Autodesk Inventor part; units mm, degrees
ref_plane "YZ Plane" through (0, 0, 0) normal (1, 0, 0) x (0, 1, 0)
ref_plane "XZ Plane" through (0, 0, 0) normal (0, 1, 0) x (-1, 0, 0)
ref_plane "XY Plane" through (0, 0, 0) normal (0, 0, 1) x (1, 0, 0)
sketch "Szkic1" plane through (0, 0, 0) normal (1, 0, 0) x (0, 1, 0)
  line L0 (0, 0) -> (50, 0)
  line L1 (50, 0) -> (50, -75)
  line L2 (50, -75) -> (0, -75)
  line L3 (0, -75) -> (0, 0)
  circle A0 centre (75, -37.5) radius 20
  line L4 (50, 0) -> (84.9897, -20.1735)
  line L5 (50, -75) -> (84.9897, -54.8265)
  dimension "d0" = 50
  dimension "d1" = 75
  dimension "d2" = 40
  dimension "d3" = 25
  dimension "d4" = 37.5
extrude "Wyciągnięcie proste1" add sketch "Szkic1" along normal blind 12
sketch "Szkic2" plane through (12, 0, 0) normal (1, 0, 0) x (0, 0, -1)
  point P0 (0, 0)
sketch "Szkic3" plane through (0, 0, 0) normal (-1, 0, 0) x (0, 0, 1)
  arc A0 (-20.1735, 84.9897) -> (-54.8265, 84.9897) centre (-37.5, 75) ccw
  circle A1 centre (-37.5, 75) radius 20
  point P0 (0, 0)
  point P1 (-54.8265, 84.9897)
  point P2 (-20.1735, 84.9897)
  dimension "d7" = 40
extrude "Wyciągnięcie proste2" add sketch "Szkic3" along normal blind 8
sketch "Szkic4" plane through (0, 0, 0) normal (-1, 0, 0) x (0, 0, 1)
  circle A0 centre (-38, 34) radius 8
  circle A1 centre (-38, 20) radius 8
  line L0 (-46, 34) -> (-46, 20)
  line L1 (-30, 34) -> (-30, 20)
  line L2 (0, 0) -> (-75, 0)
  dimension "d10" = 16
  dimension "d11" = 16
  dimension "d12" = 14
  dimension "d13" = 20
extrude "Wyciągnięcie proste3" cut sketch "Szkic4" against normal through all
sketch "Szkic5" plane through (-8, 75, -37.5) normal (-1, 0, 0) x (0, 0, 1)
  point P0 (37.5, -75)
  point P1 (0, 0)
hole "Otwór1" at (-8, 75, -37.5) direction (1, 0, 0) diameter 20 end through all
ref_plane "Płaszczyzna konstrukcyjna1" through (0, 0, -63.5) normal (0, 0, -1) x (-1, 0, 0)
sketch "Szkic6" plane through (0, 0, -63.5) normal (0, 0, -1) x (-1, 0, 0)
  circle A0 centre (20, 12.5) radius 12.5
  line L0 (0, 50) -> (-12, 50)
  line L1 (0, 50) -> (28.8115, 21.3661)
  line L2 (0, 0) -> (0, 50)
  line L3 (0, 0) -> (20, 0)
  dimension "d24" = 25
  dimension "d25" = 20
extrude "Wyciągnięcie proste4" add sketch "Szkic6" against normal blind 10
ref_plane "Płaszczyzna konstrukcyjna2" through (0, 0, -37.5) normal (0, 0, -1) x (-1, 0, 0)
sketch "Szkic7" plane through (0, 0, -63.5) normal (0, 0, -1) x (-1, 0, 0)
  arc A0 (20, 0) -> (28.8115, 21.3661) centre (20, 12.5) ccw
  circle A1 centre (20, 12.5) radius 12.5
  point P0 (0, 0)
  dimension "d28" = 25
extrude "Wyciągnięcie proste5" add sketch "Szkic7" along normal blind 2
sketch "Szkic8" plane through (-20, 12.5, -65.5) normal (0, 0, -1) x (-1, 0, 0)
  point P0 (-20, -12.5)
  point P1 (0, 0)
hole "Otwór2" at (-20, 12.5, -65.5) direction (0, 0, 1) diameter 12 end through all
mirror "Odbij1" about plane through (0, 0, -37.5) normal (0, 0, -1) of "Wyciągnięcie proste4", "Wyciągnięcie proste5", "Otwór2"
fillet "Zaokrąglenie1" radius 1 4 edges at (0, 25, -63.5) (0, 25, -21.5) (0, 25, -11.5) (0, 25, -53.5)
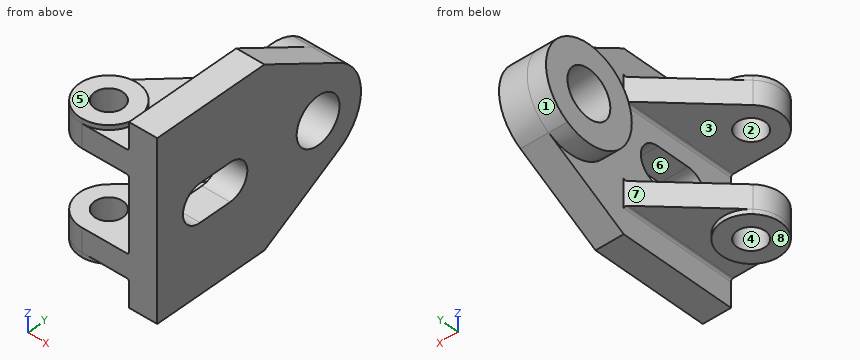
Geometry check sheet. Reference: the model listing, model coordinates, mm. Face numbers are marked on the shaded views. A direction names the side the tool comes from. Coordinates: 2 decimals unless noted, no trailing zeros. Order: outer loops, then holes, each group sorted by start corner. A loop starts at its lowest first (then second) coordinate and runs counter-clockwise, first axis right, second up. Notation, with made-up numbers: (57, 26.25) - (112, 26.25) arc R31 ccw to (112, 59.25) - close; hole circle Ø4 at (45, -39.5). An arc over 180 degrees is marked (long way). Answer in a Markdown table with one row per item. Add a question column.
1) Cross-section at C-C, the plane y = 79. Record the cut outline in (x, z).
2) Material ranges on line 1 along Y through (x, z) = (5.25, -37.5); line 2 along X through (y, z) = (12.5, -15.5); line 3 along Z through (x, y) = (8, 29.5), recorded low to high. Write a range as [from, to].
3) Cross-section at A-A, the plane z = -37.5. Record the cut outline in (x, y), then the cut area to 3 significant figures.
4) Cross-section at B-B, the plane x = -6. Record the cut outline in (y, z), then the cut area to 3 significant figures.
5) Release check for a two-part mould opening along Y. For the marked faces 1, 2, 3 and 4 record: +Y half, -Y half, draft (parallel to the pull), parting line (faces both ways), or undercut.
6) Gauge pin test, flat ends, axial feed: P1, Ø7.5, axis at x = -23.5, y = 8.5, coming from the -Z side; P2, Ø1.5, axis at x = -4.5, z = -10, coming from the -Y side; P3, Ø1.5, axis at x = -2.5, y = 27, coming from the -Z side; P4, Ø22.5, axis at y = 61.5, z = -55, coming from the -X side. Record the tip position at first contact, or that the pin passes through.
7) Cross-section at D-D, the plane x = -23. Record the cut outline in (y, z), then the cut area to 3 significant figures.
8) Set-up check for the marked faces 5, 6, 7 and 8: record each of +Z, -Z, +X, -X, +Y, -Y from which the full face is reachable in a straight line by a thin tool's end or side.
Check result:
| question | item | result |
|---|---|---|
| 1 | outline | (-8, -57.1) - (0, -57.1) - (0, -58.28) - (12, -58.28) - (12, -46.67) - (-8, -46.67) - close; (-8, -28.33) - (12, -28.33) - (12, -16.72) - (0, -16.72) - (0, -17.9) - (-8, -17.9) - close |
| 2 | line 1 | y = [0, 12.02], [41.98, 65], [85, 95] |
| 2 | line 2 | x = [-32.5, -26], [-14, 12] |
| 2 | line 3 | z = [-75, -46], [-30, 0] |
| 3 | outline | (-8, 55) - (0, 55) - (0, 41.98) - (12, 41.98) - (12, 65) - (-8, 65) - close; (-8, 85) - (12, 85) - (12, 95) - (-8, 95) - close; (0, 0) - (12, 0) - (12, 12.02) - (0, 12.02) - close |
| 3 | area | 700 mm² |
| 4 | outline | (0, -63.5) - (44.04, -63.5) - (44.04, -53.5) - (0, -53.5) - close; (0, -21.5) - (44.04, -21.5) - (44.04, -11.5) - (0, -11.5) - close; circle Ø40 at (75, -37.5); hole circle Ø20 at (75, -37.5) |
| 4 | area | 1,820 mm² |
| 5 | face 1 | +Y half |
| 5 | face 2 | undercut |
| 5 | face 3 | draft |
| 5 | face 4 | undercut |
| 6 | P1 | stops at z = -65.5 |
| 6 | P2 | passes through |
| 6 | P3 | stops at z = -63.5 |
| 6 | P4 | stops at x = -8 |
| 7 | outline | (0.37, -65.5) - (7.3, -65.5) - (7.3, -53.5) - (0.37, -53.5) - close; (0.37, -21.5) - (7.3, -21.5) - (7.3, -9.5) - (0.37, -9.5) - close; (17.7, -65.5) - (24.63, -65.5) - (24.63, -63.5) - (27.14, -63.5) - (27.14, -53.5) - (17.7, -53.5) - close; (17.7, -21.5) - (27.14, -21.5) - (27.14, -11.5) - (24.63, -11.5) - (24.63, -9.5) - (17.7, -9.5) - close |
| 7 | area | 383 mm² |
| 8 | face 5 | +Z, -X, +Y, -Y |
| 8 | face 6 | +X, -X |
| 8 | face 7 | +Z, -Z, -X |
| 8 | face 8 | -Z, -X, +Y, -Y |
